Read the model definition and answer for the solid it produces. Units are mm, in the model's axes. Face numbers are marked on the shaded views. A direction names the side the tool comes from. Coordinates: 2 decimals unless noted, no trailing zeros. Order: outer loops, then holes, each group sorted by start corner. A loop starts at its lowest first (then second) coordinate and runs counter-clockwise, first axis right, second up. Notation, with made-up numbers: M 9.5,25 L 33.5,25 A25 ccw 33.5,47 Z; hole C 53.5,86 d9. An arc over 180 degrees is marked long. Use a Markdown table: item, result. Add a question column.
1) Find section B-B on x = -35.5. Write down the section's boundary in (y, z).
2) Find section C-C on y = -22.5. Write down the section's boundary in (x, z).
3) Find the intervals of material crossed by probe 1 along X at (y, z) = (-4.5, -7); probe 2 along Z at (x, y) = (-26, -61); probe 3 along Z at (x, y) = (40, -35), in increasing order. Write a range as [from, to].
4) The mould has two halves that part along X. Classify the marked faces 1, 2 and 3: released by +X, released by -X, zero draft, split by the parting line, or undercut.
5) For the marked faces 4 and 5, determine the directions among +Z, -Z, +X, -X, +Y, -Y from which every point of the face is accessible in a straight line to the end or side of a thin tool.
6) Find section D-D on z = -31. Write down the section's boundary in (x, y), plus the area to 3 significant figures.
7) Find section A-A on z = 0. Write down the section's boundary in (x, y).
8) Each of these flat-tipped pins is pushed along its axis until it touches: pin 1 Ø2 at (x, y) = (10.5, -16) entering from -Z; pin 2 Ø5 at (y, z) = (-54, 19.5) entering from -X; pin 3 Ø10 at (x, z) = (5, 30.5) entering from +Y; pin 4 Ø15.5 at (x, y) = (36, -25) entering from +Z. Where does it stop, or does it pass through?
from build123d import *

# Parameters (mm, degrees)
F0_R     = 54.436535
F1_DEPTH = 66.294


with BuildPart() as f1:
    # F0 (on Front) → F1 (new body)
    with BuildSketch(Plane.XZ):
        Circle(F0_R)
        with BuildLine():
            ThreePointArc((-26.253978, 10.97882), (0, 28.457088), (26.253978, 10.97882))
            Line((26.253978, 10.97882), (40.456183, 10.97882))
            Line((40.456183, 10.97882), (40.456183, -10.97882))
            Line((40.456183, -10.97882), (26.253978, -10.97882))
            ThreePointArc((26.253978, -10.97882), (0, -28.457088), (-26.253978, -10.97882))
            Line((-26.253978, -10.97882), (-40.456183, -10.97882))
            Line((-40.456183, -10.97882), (-40.456183, 10.97882))
            Line((-40.456183, 10.97882), (-26.253978, 10.97882))
        make_face(mode=Mode.SUBTRACT)
    extrude(amount=F1_DEPTH)


solid = f1.part
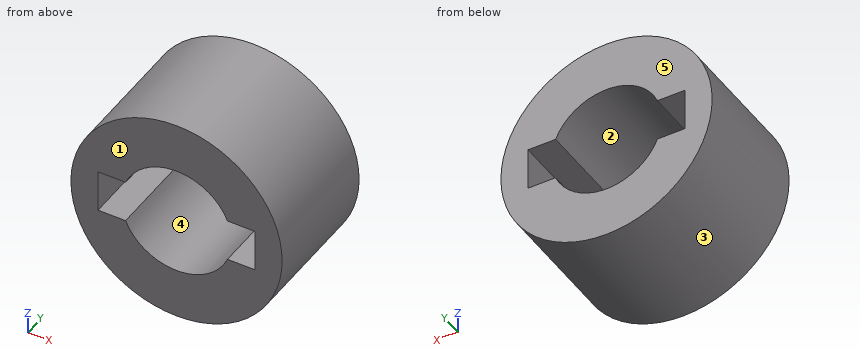
Check result:
| question | item | result |
|---|---|---|
| 1 | outline | M -66.29,-41.27 L 0,-41.27 L 0,-10.98 L -66.29,-10.98 Z; M -66.29,10.98 L 0,10.98 L 0,41.27 L -66.29,41.27 Z |
| 2 | outline | C 0,0 d108.87; hole M -40.46,-10.98 L -26.25,-10.98 A28.46 ccw 26.25,-10.98 L 40.46,-10.98 L 40.46,10.98 L 26.25,10.98 A28.46 ccw -26.25,10.98 L -40.46,10.98 Z |
| 3 | probe 1 | x = [-53.98, -40.46], [40.46, 53.98] |
| 3 | probe 2 | z = [-47.83, -11.57], [11.57, 47.83] |
| 3 | probe 3 | z = [-36.92, -10.98], [10.98, 36.92] |
| 4 | face 1 | zero draft |
| 4 | face 2 | undercut |
| 4 | face 3 | split by the parting line |
| 5 | face 4 | +Y, -Y |
| 5 | face 5 | +Z, -Z, +X, -X, +Y |
| 6 | outline | M -44.75,-66.29 L 44.75,-66.29 L 44.75,0 L -44.75,0 Z |
| 6 | area | 5,930 mm2 |
| 7 | outline | M -54.44,-66.29 L -40.46,-66.29 L -40.46,0 L -54.44,0 Z; M 40.46,-66.29 L 54.44,-66.29 L 54.44,0 L 40.46,0 Z |
| 8 | pin 1 | stops at z = -53.6 |
| 8 | pin 2 | stops at x = -51.71 |
| 8 | pin 3 | stops at y = 0 |
| 8 | pin 4 | stops at z = 46.53 |
